Design review of the part built by this model. Coordinates are the model's own, in mm. Face numbers are marked on the shaded views. A direction names the side the tool comes from. Coordinates: 2 decimals unless noted, no trailing zeros. Loops run counter-clockwise (first coordinate to the right, second up) from the corner with the lowest first, then second, coordinate; pieces in that order, holes last. Notation, with made-up numbers: (2.25, 60.25) -> (56.25, 60.25) arc R16 ccw to (56.25, 79.25) -> close; hole circle Ø3 at (-24, -7). An arc over 180 degrees is marked (long way). One line per item, written item: value. Start each with the question number.
1. Add section A-A on y = 23. Write out the cut boundary in (x, z).
2. Machinability: for the marked faces 1 and 2, which of the approach directions +Z, -Z, +X, -X, +Y, -Y give a long, thin tool a straight path to every point of the face, cutting with its end or side? Answer none if there is none.
3. Insertion check: pin 1 (8 mm diameter, centred on x = 79, z = -22, fed in from +Y). The pin has a flat end and moves straight along its axis. Give the tip position at first contact, or say it passes through.
4. Add section C-C on x = 133.5. Write out the cut boundary in (y, z), plus the area to 3 significant figures.
5. For probe 1 along X at (y, z) = (46, -39); probe 2 along Z at (x, y) = (81, 18.5); probe 3 along Y at (x, z) = (9.5, -44), list the stretches that pass through material, from the lowest coordinate up.
6. Add section B-B on z = -15.5. Write out the cut boundary in (x, y).
7. Draft analysis for pull direction X (two halves, no side actions). For the marked faces 3, 4 and 5, state which applies: pulls with the +X half, pulls with the -X half, needs draft (parallel to the pull), parting line crosses it, or undercut.
```python
from build123d import *

# Parameters (mm, degrees)
EXTRUDE_1_DEPTH = 50
SHELL_1_T       = -1.6


with BuildPart() as part:
    # 草图1 → 凸台-拉伸1 (new body)
    with BuildSketch(Plane(origin=(0, 0, 0), x_dir=(1, 0, 0), z_dir=(0, 1, 0))):
        with BuildLine():
            Line((10, 0), (140, 0))
            ThreePointArc((140, 0), (147.071067812, 2.928932188), (150, 10))
            Line((150, 10), (150, 40))
            ThreePointArc((150, 40), (147.071067812, 47.071067812), (140, 50))
            Line((140, 50), (10, 50))
            ThreePointArc((10, 50), (2.928932188, 47.071067812), (0, 40))
            Line((0, 40), (0, 10))
            ThreePointArc((0, 10), (2.928932188, 2.928932188), (10, 0))
        make_face()
    extrude(amount=EXTRUDE_1_DEPTH)

    # 抽壳1
    shell_1_openings = [part.faces().sort_by_distance(p)[0] for p in [
        (75, 50, -25),
    ]]
    offset(amount=SHELL_1_T, openings=shell_1_openings, kind=Kind.INTERSECTION)


solid = part.part
```
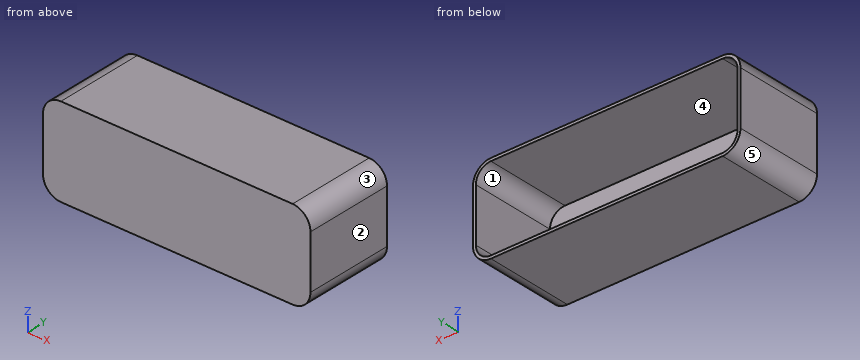
Worked answers:
1. outline: (0, -40) arc R10 ccw to (10, -50) -> (140, -50) arc R10 ccw to (150, -40) -> (150, -10) arc R10 ccw to (140, 0) -> (10, 0) arc R10 ccw to (0, -10) -> close; hole (1.6, -40) arc R8.4 ccw to (10, -48.4) -> (140, -48.4) arc R8.4 ccw to (148.4, -40) -> (148.4, -10) arc R8.4 ccw to (140, -1.6) -> (10, -1.6) arc R8.4 ccw to (1.6, -10) -> close
2. face 1: +Y
2. face 2: +Z, -Z, +X, +Y, -Y
3. pin 1: stops at y = 1.6
4. outline: (0, -50) -> (50, -50) -> (50, -48.4) -> (1.6, -48.4) -> (1.6, -1.6) -> (50, -1.6) -> (50, 0) -> (0, 0) -> close
4. area: 235 mm²
5. probe 1: x = 0 to 1.6, 148.4 to 150
5. probe 2: z = -50 to -48.4, -1.6 to 0
5. probe 3: y = 0 to 1.6
6. outline: (0, 0) -> (150, 0) -> (150, 50) -> (148.4, 50) -> (148.4, 1.6) -> (1.6, 1.6) -> (1.6, 50) -> (0, 50) -> close
7. face 3: pulls with the +X half
7. face 4: undercut
7. face 5: pulls with the -X half
